Input: part model. Units: mm. Frame: model coordinates. A direction names the side the tool comes from. Round coordinates to 2 decimals unless told otherwise and drop trailing zeros. Loops run counter-clockwise (first coordinate to the right, second up) from the corner with the lowest first, then second, coordinate; pieces in that order, holes last. Notation, with made-up numbers: M -18,58 L 32,58 A18 cw 32,81 Z; hole C 73,-17.75 d5. An arc over 180 degrees is marked long. Return JSON: item names as keys, results as strings. Group by question number.
1) Access query for faces 5 (the face through (8, 0, 2)), 6 (the face through (11.423, 6.622, 1.726)), 7 (the face through (4.5, 8.5, 4.5)). Directions: +Z, -Z, +X, -X, +Y, -Y. A direction counts if a zero-diameter tool reaches every point of the face in a straight line with its end or side. Return the directions, or none.
2) Mould query, pull axis Y, two halves, no side actions, for faces 1 (the face through (10.13, 5.073, 5.018)), 2 (the face through (0, 8, 2)), 3 (the face through (8, 16.8, 2)), 4 (the face through (6.8, 7.2, 4.6)). Classes: +Y half, -Y half, draft (parallel to the pull), parting line (faces both ways), or undercut.
3) Contact query for a flat-ended pin moving along its axis: P1, Ø6.5, axis at x = 8.4, y = 8.4, coming from the -Z side. Output: stop coordinate, or through.
4) Material intervals for line 1 (Y direction, x = 8.4, z = 4.8); line 2 (X direction, y = 8.4, z = 4.15), sorted ascending. Write a range as from..to.
5) Section A-A (x = 8.4). Output: boundary loops of the cut face in (y, z), plus the area to 3 significant figures.
6) Section C-C (y = 13). Output: boundary loops of the cut face in (x, z).
7) Section B-B (z = 1.5). Output: boundary loops of the cut face in (x, y) (3 decimals), plus the area to 3 significant figures.
from build123d import *

# Parameters (mm, degrees)
SKETCH_W      = 16.8
SKETCH_H      = 16.8
SKETCH_R      = 2
PAD_DEPTH     = 4.5
SKETCH002_R   = 3.75
SKETCH002_R_2 = 2
PAD001_DEPTH  = 1.3
POCKET_DEPTH  = 3.5
FILLET_R      = 0.25


with BuildPart() as part:
    # Sketch → Pad (new body)
    with BuildSketch(Plane.XY):
        with Locations((8.4, 8.4)):
            Rectangle(SKETCH_W, SKETCH_H)
        with Locations((8.4, 8.4)):
            Circle(SKETCH_R, mode=Mode.SUBTRACT)
    extrude(amount=PAD_DEPTH)

    # Sketch002 (on Face7 of Pad) → Pad001 (join)
    with BuildSketch(Plane.XY.offset(4.5)):
        with Locations((8.4, 8.4)):
            Circle(SKETCH002_R)
        with Locations((8.4, 8.4)):
            Circle(SKETCH002_R_2, mode=Mode.SUBTRACT)
    extrude(amount=PAD001_DEPTH)

    # Sketch001 → Pocket (cut)
    with BuildSketch(Plane.XY):
        Polygon((12.45, 8.4), (10.425, 11.907403), (6.375, 11.907403), (4.35, 8.4), (6.375, 4.892597), (10.425, 4.892597), align=None)
    extrude(amount=POCKET_DEPTH, mode=Mode.SUBTRACT)

    # Fillet
    fillet_edges = [part.edges().sort_by_distance(p)[0] for p in [
        (4.65, 8.4, 5.8),
    ]]
    fillet(fillet_edges, radius=FILLET_R)


solid = part.part
Returned:
{
 "1": {"face 5": "+Z, -Z, +X, -X, -Y", "face 6": "-Z", "face 7": "+Z"},
 "2": {"face 1": "parting line", "face 2": "draft", "face 3": "+Y half", "face 4": "undercut"},
 "3": {"P1": "stops at z = 3.5"},
 "4": {"line 1": "y = 4.65..6.4, 10.4..12.15", "line 2": "x = 0..6.4, 10.4..16.8"},
 "5": {"outline": "M 0,0 L 4.89,0 L 4.89,3.5 L 6.4,3.5 L 6.4,5.8 L 4.9,5.8 A0.25 ccw 4.65,5.55 L 4.65,4.5 L 0,4.5 Z; M 10.4,3.5 L 11.91,3.5 L 11.91,0 L 16.8,0 L 16.8,4.5 L 12.15,4.5 L 12.15,5.55 A0.25 ccw 11.9,5.8 L 10.4,5.8 Z", "area": "51.6 mm^2"},
 "6": {"outline": "M 0,0 L 16.8,0 L 16.8,4.5 L 0,4.5 Z"},
 "7": {"outline": "M 0,0 L 16.8,0 L 16.8,16.8 L 0,16.8 Z; hole M 4.35,8.4 L 6.375,4.893 L 10.425,4.893 L 12.45,8.4 L 10.425,11.907 L 6.375,11.907 Z", "area": "240 mm^2"}
}
